Can you work these out from the model? Positions are in its coordinate system, mm. Face numbers are marked on the shaded views. A direction names the side the tool comes from. Coordinates: 2 decimals unless noted, no trailing zeros. Order: outer loops, then holes, each group sorted by start corner. A loop starts at its lowest first (then second) coordinate and runs counter-clockwise, first axis right, second up. Notation, with made-up numbers: (39, 83.5) -> (89, 83.5) arc R18 ccw to (89, 111.5) -> close; hole circle Ø8 at (87.5, 86.5). An arc over 180 degrees is marked (long way). Answer in a Markdown table with one row per item. Add a question column.
1. Imagine slicing it at D-D on x = 30. Write out the boundary of the cut face in (y, z), plus the area to 3 significant figures.
2. On a 3-axis mill with a long thin cutter (end or side, diameter ignored), from which of +Z, -Z, +X, -X, +Y, -Y can I reach the whole of each face in a straight line? I mean the marked faces 1, 2 and 3. Say none if no direction works.
3. Imagine slicing it at A-A on y = 13. Write out the boundary of the cut face in (x, z).
4. We'd pull the mould along Z, two halves only. Please class the marked faces 4, 5, 6 and 7: pulls with the +Z half, pulls with the -Z half, needs draft (parallel to the pull), parting line crosses it, or undercut.
5. If I drill on line 1 along Y through (x, z) = (30, 16.5); line 2 along Y through (x, z) = (29, 7.25); line 3 along Z through (x, y) = (28, 21), over which ranges is the centre line in solid material (lowest first)? Write a range as [from, to].
6. Imagine slicing it at C-C on y = 90. Write out the boundary of the cut face in (x, z).
7. Will these pins go through, and if not, where does the flat tip stop? pin 1 (8 mm diameter, centred on x = 51, y = 55.5, fed in from +Z); pin 2 (8 mm diameter, centred on y = 84.5, z = 9, fed in from +X); pin 3 (0.8 mm diameter, centred on x = 36.5, z = 16.5, fed in from +Y).
8. Imagine slicing it at B-B on z = 11.75. Write out the boundary of the cut face in (x, y).
from build123d import *

# Parameters (mm, degrees)
F0_W     = 60
F0_H     = 90
F1_DEPTH = 20
F2_R     = 49.5
F3_DEPTH = 20
F4_R     = 47
F5_DEPTH = 17
F8_DEPTH = 79.501


with BuildPart() as f1:
    # F0 (on Top) → F1 (new body)
    with BuildSketch(Plane.XY):
        with Locations((30, 45)):
            Rectangle(F0_W, F0_H)
    extrude(amount=F1_DEPTH)

    # F2 (on Top) → F3 (join)
    with BuildSketch(Plane.XY):
        with Locations((30, 90)):
            Circle(F2_R)
    extrude(amount=F3_DEPTH)

    # F4 (on face) → F5 (cut)
    with BuildSketch(Plane.XY.offset(20)):
        with Locations((30, 90)):
            Circle(F4_R)
    extrude(amount=-F5_DEPTH, mode=Mode.SUBTRACT)

    # F7 (on face) → F8 (cut, through all)
    with BuildSketch(Plane.YZ.offset(60)):
        Polygon((11.123074, 16), (0, 16), (0, 4), (17.377608, 4), (38, 4), (38, 16), (38, 17), (11.123074, 17), align=None)
    extrude(amount=-F8_DEPTH, mode=Mode.SUBTRACT)


solid = f1.part
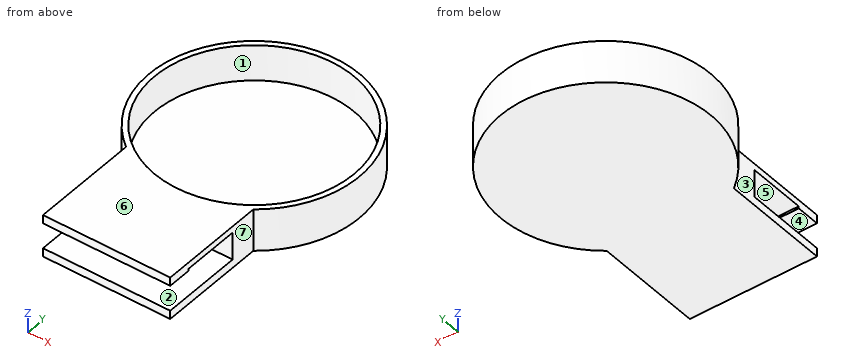
Answers follow:
| question | item | result |
|---|---|---|
| 1 | outline | (0, 0) -> (139.5, 0) -> (139.5, 20) -> (137, 20) -> (137, 3) -> (43, 3) -> (43, 20) -> (0, 20) -> (0, 16) -> (11.12, 16) -> (11.12, 17) -> (38, 17) -> (38, 4) -> (0, 4) -> close |
| 1 | area | 709 mm² |
| 2 | face 1 | +Z |
| 2 | face 2 | +X, -X, -Y |
| 2 | face 3 | +Z, -Z, -X, -Y |
| 3 | outline | (0, 0) -> (60, 0) -> (60, 4) -> (0, 4) -> close; (0, 17) -> (60, 17) -> (60, 20) -> (0, 20) -> close |
| 4 | face 4 | undercut |
| 4 | face 5 | undercut |
| 4 | face 6 | pulls with the +Z half |
| 4 | face 7 | needs draft |
| 5 | line 1 | y = [0, 11.12], [38, 43], [137, 139.5] |
| 5 | line 2 | y = [38, 43.01], [136.99, 139.49] |
| 5 | line 3 | z = [0, 4], [17, 20] |
| 6 | outline | (-19.5, 0) -> (79.5, 0) -> (79.5, 20) -> (77, 20) -> (77, 3) -> (-17, 3) -> (-17, 20) -> (-19.5, 20) -> close |
| 7 | pin 1 | stops at z = 3 |
| 7 | pin 2 | stops at x = 79.48 |
| 7 | pin 3 | stops at y = 139.12 |
| 8 | outline | (0, 38) -> (60, 38) -> (60, 50.63) arc R49.5 ccw (long way) to (0, 50.63) -> close; hole circle Ø94 at (30, 90) |
